Here's the drawing with two shaded views (mm, measured from the low corner). I have some questions. Coordinates: 2 decimals unless noted, no trailing zeros. Order: outer loops, then holes, each group sorted by start corner. A loop starts at its lowest first (then second) coordinate and runs counter-clockwise, first axis right, second up. Notation, with made-up numbers: (-28.5, 59) -> (-14.5, 59) arc R26 cw to (-14.5, 95) -> close; hole circle Ø1 at (3.5, 72). An arc over 180 degrees is marked (long way). Write item = value, one per line.
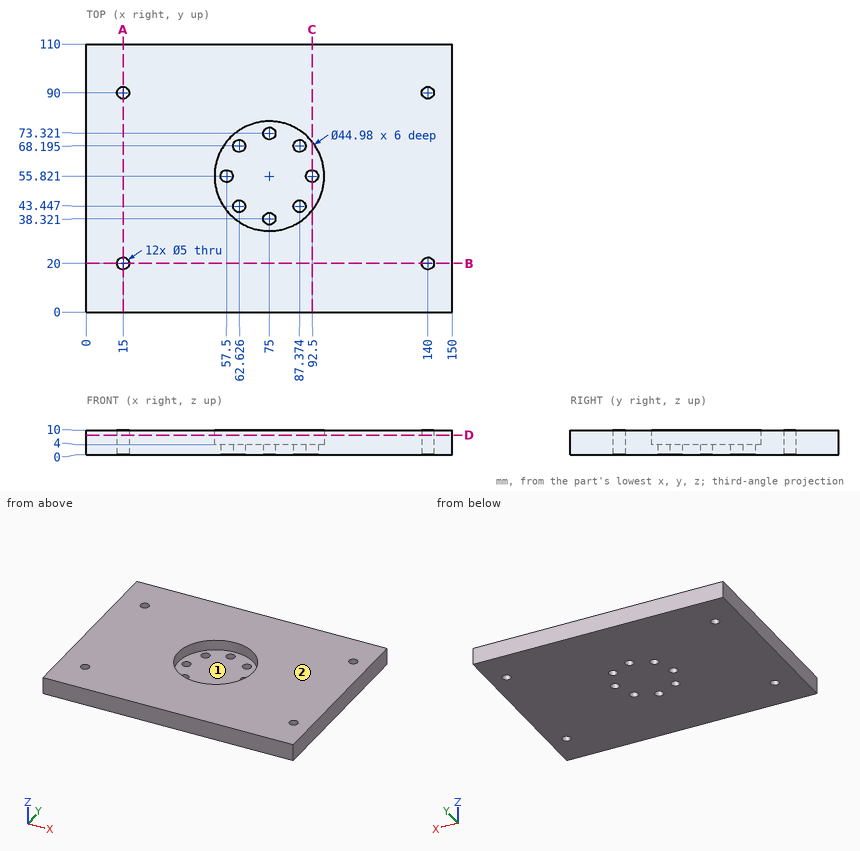
Item 1: If we mould it in two halves opening along X, with no side actions, what happens to the marked faces 1 and 2? For each: pulls with the +X half, pulls with the -X half, needs draft (parallel to the pull), parting line crosses it, or undercut.
A:
face_1 = undercut
face_2 = needs draft
Item 2: I want a section at B-B, the plane y = 20. Please give me the cut outline in (x, z).
A:
outline = (0, 0) -> (12.5, 0) -> (12.5, 10) -> (0, 10) -> close; (17.5, 0) -> (137.5, 0) -> (137.5, 10) -> (17.5, 10) -> close; (142.5, 0) -> (150, 0) -> (150, 10) -> (142.5, 10) -> close
Item 3: I want a section at D-D, the plane z = 8. Please give me the cut outline in (x, y).
A:
outline = (0, 0) -> (150, 0) -> (150, 110) -> (0, 110) -> close; hole circle Ø5 at (15, 20); hole circle Ø5 at (15, 90); hole circle Ø44.98 at (75, 55.82); hole circle Ø5 at (140, 20); hole circle Ø5 at (140, 90)
Item 4: I want a section at A-A, the plane x = 15. Please give me the cut outline in (y, z).
A:
outline = (0, 0) -> (17.5, 0) -> (17.5, 10) -> (0, 10) -> close; (22.5, 0) -> (87.5, 0) -> (87.5, 10) -> (22.5, 10) -> close; (92.5, 0) -> (110, 0) -> (110, 10) -> (92.5, 10) -> close
Item 5: If I drill on probe 1 along Y at (x, z) = (92.5, 2.65); probe 2 along Y at (x, z) = (141, 0.5); probe 3 along Y at (x, z) = (89, 2) (1 decimal), over which ranges is the centre line in solid material (lowest first)?
A:
probe_1 = 0 to 53.32, 58.32 to 110
probe_2 = 0 to 17.71, 22.29 to 87.71, 92.29 to 110
probe_3 = 0 to 41.5, 45.3 to 66.3, 70.1 to 110
Item 6: I want a section at C-C, the plane x = 92.5. Please give me the cut outline in (y, z) (1 decimal).
A:
outline = (0, 0) -> (53.3, 0) -> (53.3, 4) -> (41.7, 4) -> (41.7, 10) -> (0, 10) -> close; (58.3, 0) -> (110, 0) -> (110, 10) -> (69.9, 10) -> (69.9, 4) -> (58.3, 4) -> close
Item 7: I'm going to push a flat-ended pin straight in: P1, Ø6.5, axis at x = 87.37, y = 68.2, coming from the +Z side. Where does the tip first touch, or does it pass through?
A:
P1 = 4
